Design review of the part built by this model. Coordinates are the model's own, in mm. Face numbers are marked on the shaded views. A direction names the side the tool comes from. Give positions to 0.01 mm unless a question says otherwise; leave off trailing zeros. Loops run counter-clockwise (first coordinate to the right, second up) from the corner with the lowest first, then second, coordinate; pieces in that order, holes last. Notation, with made-up numbers: (49.25, -24) - (89.25, -24) arc R31 cw to (89.25, 8) - close; hole circle Ø1 at (72, 20). An arc over 180 degrees is marked (long way). Write each question's results on one line, items separated by ' | '.
Autodesk Inventor part; units mm, degrees
ref_plane "YZ Plane" through (0, 0, 0) normal (1, 0, 0) x (0, 1, 0)
ref_plane "XZ Plane" through (0, 0, 0) normal (0, 1, 0) x (-1, 0, 0)
ref_plane "XY Plane" through (0, 0, 0) normal (0, 0, 1) x (1, 0, 0)
sketch "Sketch1" plane through (0, 0, 0) normal (0, 0, 1) x (1, 0, 0)
  line L0 (-17, 28) -> (0, 28)
  line L1 (0, 28) -> (0, 0)
  line L2 (0, 0) -> (-17, 0)
  line L3 (-17, 0) -> (-17, 28)
  dimension "d0" = 17
  dimension "d1" = 28
extrude "Extrusion1" add sketch "Sketch1" along normal blind 1
sketch "Sketch2" plane through (0, 0, 1) normal (0, 0, 1) x (1, 0, 0)
  line L0 (-17, 28) -> (-17, 0)
  line L1 (0, 28) -> (-17, 28)
  line L2 (0, 0) -> (0, 28)
  line L3 (-17, 0) -> (0, 0)
  circle A0 centre (-12.5, 26) radius 1.35
  circle A1 centre (-4.5, 5) radius 1.35
  dimension "d4" = 2.7
  dimension "d5" = 2.7
  dimension "d6" = 4.5
  dimension "d7" = 4.5
  dimension "d8" = 2
  dimension "d9" = 5
extrude "Extrusion2" cut sketch "Sketch2" against normal through all contours A0 | A1
sketch "Sketch3" plane through (0, 0, 1) normal (0, 0, 1) x (1, 0, 0)
  circle A0 centre (-12.5, 26) radius 1.35
  circle A1 centre (-4.5, 5) radius 1.35
  line L0 (0, 28) -> (-17, 28)
  line L1 (-17, 28) -> (-17, 0)
  line L2 (-17, 0) -> (0, 0)
  line L3 (0, 0) -> (0, 28)
  circle A2 centre (-8.5, 12.047) radius 6.5
  dimension "d12" = 13
  dimension "d13" = 12.047
extrude "Extrusion3" add sketch "Sketch3" along normal blind 30 contours A2
sketch "Sketch4" plane through (-8.5, 12.047, 31) normal (0, 0, 1) x (1, 0, 0)
  circle A0 centre (0, 0) radius 6.5
  circle A1 centre (0, 0) radius 3.5
  point P0 (8.5, -12.047)
  dimension "d16" = 7
sketch "Sketch5" plane through (0, 0, 0) normal (0, 0, -1) x (-1, 0, 0)
  circle A0 centre (8.5, 12.047) radius 6.5
  circle A1 centre (8.5, 12.047) radius 5
  point P0 (0, 0)
  dimension "d17" = 10
loft "Loft1" cut profiles "Sketch5", "Sketch4" contours A1 / A1
sketch "Sketch6" plane through (-8.5, 12.047, 31) normal (0, 0, 1) x (1, 0, 0)
  circle A0 centre (0, 0) radius 3.5
  circle A1 centre (0, 0) radius 4.75
  point P0 (8.5, -12.047)
  dimension "d26" = 9.5
extrude "Extrusion6" add sketch "Sketch6" along normal blind 3
sketch "Sketch7" plane through (-8.5, 12.047, 34) normal (0, 0, 1) x (1, 0, 0)
  circle A0 centre (0, 0) radius 3.5
  circle A1 centre (0, 0) radius 4.75
  line L0 (2, 0) -> (-2, 0)
  line L1 (-2, 0) -> (-2, 6)
  line L2 (-2, 6) -> (2, 6)
  line L3 (2, 6) -> (2, 0)
  point P0 (8.5, -12.047)
  dimension "d29" = 4
  dimension "d30" = 2
extrude "Extrusion7" cut sketch "Sketch7" against normal up to surface (3 mm away) contours L3 L0 L1 A0 | A0 L1 A1 L3 | A1 L1 L2 L3 picked at (0.1416, 1.158) picked at (-1.4244, 4.0721)
properties part number "TORRE"
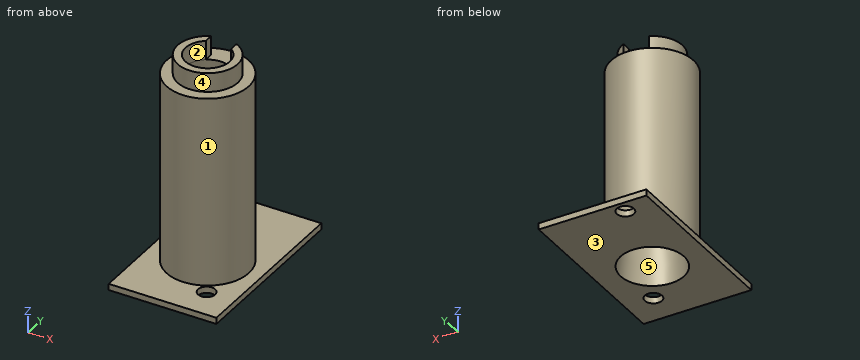
Item 1: We need section A-A on y = 5. Give the boundary of the cut face in (x, z), then the cut area to 3 significant figures.
Output values:
outline: (-17, 0) - (-5.85, 0) - (-5.85, 1) - (-17, 1) - close; (-3.15, 0) - (0, 0) - (0, 1) - (-3.15, 1) - close | area: 14.3 mm²
Item 2: Draft analysis for pull direction X (two halves, no side actions). For the marked faces 1, 2 and 3, state which applies: +X half, -X half, draft (parallel to the pull), parting line (faces both ways), or undercut.
Output values:
face 1: parting line | face 2: undercut | face 3: draft
Item 3: We need section B-B on x = -15.5. Give the boundary of the cut face in (y, z).
Output values:
outline: (0, 0) - (28, 0) - (28, 1) - (0, 1) - close
Item 4: Wall thickness on probe 1 along Y at (x, z) = (-12.5, 0.75); probe 2 along Z at (x, y) = (-0.75, 22.25); probe 3 along Z at (x, y) = (-6, 7): over which ranges is each line inside the solid? List them lowest first.
Output values:
probe 1: y = 0 to 9.11, 14.99 to 24.65, 27.35 to 28 | probe 2: z = 0 to 1 | probe 3: z = 0 to 31
Item 5: We need section C-C on z = 17.5. Give the boundary of the cut face in (x, y), then the cut area to 3 significant figures.
Output values:
outline: circle Ø13 at (-8.5, 12.05); hole circle Ø8.31 at (-8.5, 12.05) | area: 78.5 mm²
Item 6: We need section D-D on y = 23. Give the boundary of the cut face in (x, z).
Output values:
outline: (-17, 0) - (0, 0) - (0, 1) - (-17, 1) - close
Item 7: Tool access review of the marked faces 4 and 5: name each direction out of +Z, -Z, +X, -X, +Y, -Y from which nothing blocks a thin tool from reaching the whole face with its end or side.
Output values:
face 4: +Z | face 5: -Z
Item 8: Clearance check with flat-ended pins moving along their axes: P1, Ø3, axis at x = -4.5, y = 5, coming from the -Z side; P2, Ø1.6, axis at y = 16, z = 32, coming from the +X side; P3, Ø10, axis at x = -14, z = 21.5, coming from the +Y side; P4, Ø12, axis at y = 21.5, z = 12.5, coming from the +X side. State where each tip first meets the part, or that it passes through.
Output values:
P1: stops at z = 0 | P2: stops at x = -4.95 | P3: stops at y = 18.53 | P4: stops at x = -2.99
